Geometry check sheet. Reference: the model listing, model coordinates, mm. Give positions to 0.01 mm unless a question says otherwise; leave off trailing zeros. Write each loop counter-clockwise with the first axis right and the second up, starting at its lowest first coordinate (ties: lowest second). Pieces come first, ordered by that corner, then holes. Notation, with made-up numbers: (-32.5, 5.5) - (15.5, 5.5) arc R34 cw to (15.5, 36.5) - close; hole circle Ø5 at (17.5, 29). An arc over 180 degrees is marked (long way). Use a Markdown table: item, result.
Autodesk Inventor part; units mm, degrees
ref_plane "YZ Plane" through (0, 0, 0) normal (1, 0, 0) x (0, 1, 0)
ref_plane "XZ Plane" through (0, 0, 0) normal (0, 1, 0) x (-1, 0, 0)
ref_plane "XY Plane" through (0, 0, 0) normal (0, 0, 1) x (1, 0, 0)
sketch "Boceto1" plane through (0, 0, 0) normal (1, 0, 0) x (0, 1, 0)
  circle A0 centre (0, 0) radius 25
  line L0 (35, 43.3169) -> (35, 40)
  line L1 (-35, 43.3169) -> (-35, 40)
  line L2 (35, -40) -> (35, -43.3169)
  line L3 (-35, -40) -> (-35, -43.3169)
  arc A1 (33.3333, 45.289) -> (-33.3333, 45.289) centre (0, -151.9137) ccw
  arc A2 (-33.3333, -45.289) -> (33.3333, -45.289) centre (0, 151.9137) ccw
  arc A3 (-24.0379, 6.8686) -> (-35, 40) centre (-53.845, 15.3856) ccw
  arc A4 (-35, -40) -> (-24.0379, -6.8686) centre (-53.845, -15.3856) ccw
  arc A5 (35, 40) -> (24.9998, -0.1114) centre (111.9989, -0.499) ccw
  arc A6 (24.9998, 0.1114) -> (35, -40) centre (111.9989, 0.499) ccw
  arc A7 (35, 43.3169) -> (33.3333, 45.289) centre (33, 43.3169) ccw
  arc A8 (-33.3333, 45.289) -> (-35, 43.3169) centre (-33, 43.3169) ccw
  arc A9 (33.3333, -45.289) -> (35, -43.3169) centre (33, -43.3169) ccw
  arc A10 (-35, -43.3169) -> (-33.3333, -45.289) centre (-33, -43.3169) ccw
  point P0 (35, 45)
  point P1 (-35, 45)
  point P2 (35, -45)
  point P3 (-35, -45)
  dimension "d0" = 50
  dimension "d1" = 5
  dimension "d2" = 70
  dimension "d3" = 35
  dimension "d4" = 0
  dimension "d5" = 70
  dimension "d6" = 0
  dimension "d8" = 40
  dimension "d9" = 40
  dimension "d10" = 200
  dimension "d12" = 200
  dimension "d13" = 31
  dimension "d14" = 31
  dimension "d15" = 87
  dimension "d17" = 87
  dimension "d20" = 2
  dimension "d21" = 2
  dimension "d22" = 2
extrude "Extrusión1" add sketch "Boceto1" along normal blind 3.3
sketch "Boceto2" plane through (3.3, 0, 0) normal (1, 0, 0) x (0, 0, -1)
  arc A0 (-40, 35) -> (0, 25.0003) centre (0.499, 111.9989) ccw
  arc A1 (40, -35) -> (6.8686, -24.0379) centre (15.3856, -53.845) ccw
  arc A2 (0, 25.0003) -> (40, 35) centre (-0.499, 111.9989) ccw
  arc A3 (-6.8686, -24.0379) -> (-40, -35) centre (-15.3856, -53.845) ccw
  line L0 (-40, 35) -> (-43.3, 35)
  line L1 (-43.3, 35) -> (-43.3, 24)
  line L2 (-43.3, 24) -> (-40, 24)
  line L3 (-40, 24) -> (-40, 35)
  line L4 (-40, -35) -> (-43.3, -35)
  line L5 (-43.3, -35) -> (-43.3, -30)
  line L6 (-43.3, -30) -> (-40, -30)
  line L7 (-40, -30) -> (-40, -35)
  line L8 (40, 35) -> (43.3, 35)
  line L9 (43.3, 35) -> (43.3, 24)
  line L10 (43.3, 24) -> (40, 24)
  line L11 (40, 24) -> (40, 35)
  line L12 (40, -35) -> (43.3, -35)
  line L13 (43.3, -35) -> (43.3, -30)
  line L14 (43.3, -30) -> (40, -30)
  line L15 (40, -30) -> (40, -35)
  circle A4 centre (0, 0) radius 20
  line L16 (-41, 18) -> (-25, 18)
  line L17 (-25, 18) -> (-25, 5)
  line L18 (-25, 5) -> (-41, 5)
  line L19 (-41, 5) -> (-41, 18)
  line L20 (-41, -5) -> (-25, -5)
  line L21 (-25, -5) -> (-25, -18)
  line L22 (-25, -18) -> (-41, -18)
  line L23 (-41, -18) -> (-41, -5)
  line L24 (25, 18) -> (41, 18)
  line L25 (41, 18) -> (41, 5)
  line L26 (41, 5) -> (25, 5)
  line L27 (25, 5) -> (25, 18)
  line L28 (25, -5) -> (41, -5)
  line L29 (41, -5) -> (41, -18)
  line L30 (41, -18) -> (25, -18)
  line L31 (25, -18) -> (25, -5)
  point P0 (-6.2262, 34.4418)
  point P1 (12.6899, -32.6185)
  point P2 (6.2262, 34.4418)
  dimension "d31" = 40
  dimension "d23" = 3.3
  dimension "d24" = 3.3
  dimension "d25" = 3.3
  dimension "d26" = 3.3
  dimension "d27" = 11
  dimension "d28" = 5
  dimension "d34" = 16
  dimension "d35" = 13
  dimension "d37" = 25
  dimension "d38" = 5
  dimension "d40" = 5
  dimension "d41" = 25
extrude "Extrusión2" cut sketch "Boceto2" against normal blind 3.3
equation "\"d5\" = d2"
equation "\"d14\" = d13"
equation "\"d17\" = d15"
equation "\"d25\" = d23"
equation "\"Radio_pliegue\" = Grosor"
equation "\"Anchura_desahogo_plegado\" = Grosor"
equation "\"Profundidad_desahogo_plegado\" = 0.5 * Grosor"
equation "\"Tamaño_destalonado\" = 4 * Grosor"
equation "\"Remanente_mínimo\" = 2 * Grosor"
equation "\"Radiodetransición\" = Radio_pliegue"
equation "\"Tamaño_de_radio_de_Jacobi\" = Grosor"
equation "\"TamañoSeparación\" = Grosor"
properties part number "Cuerpo - Unión Laterales"
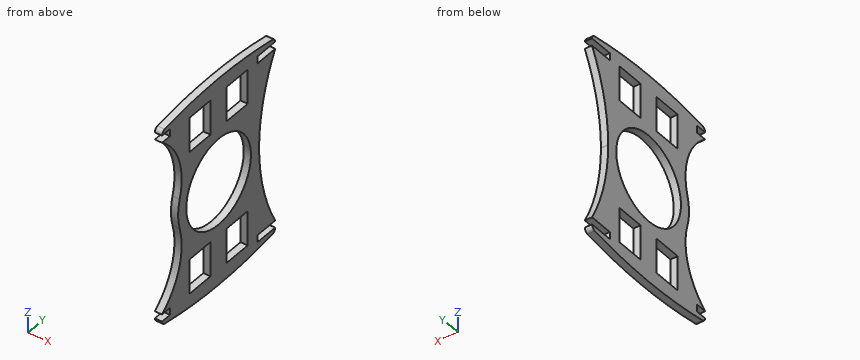
1) Section check D-D on z = -37. Record the boundary of the cut face in (x, y), then the cut area to 3 significant figures.
Working result:
| item | result |
|---|---|
| outline | (0, -31.62) - (3.3, -31.62) - (3.3, -18) - (0, -18) - close; (0, -5) - (3.3, -5) - (3.3, 5) - (0, 5) - close; (0, 18) - (3.3, 18) - (3.3, 33.5) - (0, 33.5) - close |
| area | 129 mm² |
2) Section check B-B on z = 29. Record the boundary of the cut face in (x, y).
Working result:
| item | result |
|---|---|
| outline | (0, -25.99) - (3.3, -25.99) - (3.3, -18) - (0, -18) - close; (0, -5) - (3.3, -5) - (3.3, 5) - (0, 5) - close; (0, 18) - (3.3, 18) - (3.3, 30.15) - (0, 30.15) - close |
3) Section check A-A on y = 0. Record the boundary of the cut face in (x, z).
Working result:
| item | result |
|---|---|
| outline | (0, -48.09) - (3.3, -48.09) - (3.3, -20) - (0, -20) - close; (0, 20) - (3.3, 20) - (3.3, 48.09) - (0, 48.09) - close |
4) Depth check by flat-ended pin: P1, Ø1.6, axis at x = 1.5, z = 41.5, coming from the +Y side; P2, Ø1.6, axis at x = 1.5, z = 34, coming from the +Y side; P3, Ø1, axis at x = 1.5, y = 31.5, coming from the +Z side. Enter the tip coordinate at first touch or a pass-through.
Working result:
| item | result |
|---|---|
| P1 | stops at y = 24 |
| P2 | stops at y = 32.48 |
| P3 | stops at z = 45.67 |
5) Material ranges on L1, parallel to Z at x = 0.1, y = -8; L2, parallel to Y at x = 2.4, z = 34; L3, parallel to Y at x = 0.4, z = 27.5, recorded low to high. Write a range as from..to.
Working result:
| item | result |
|---|---|
| L1 | z = -47.93..-41, -25..-18.33, 18.33..25, 41..47.93 |
| L2 | y = -29.06..-18, -5..5, 18..32.13 |
| L3 | y = -25.31..-18, -5..5, 18..29.63 |
6) Section check C-C on z = -17. Record the boundary of the cut face in (x, y), then the cut area to 3 significant figures.
Working result:
| item | result |
|---|---|
| outline | (0, -22.89) - (3.3, -22.89) - (3.3, -10.54) - (0, -10.54) - close; (0, 10.54) - (3.3, 10.54) - (3.3, 26.78) - (0, 26.78) - close |
| area | 94.4 mm² |
